The listing builds one solid part. Answer for the finished solid, in the listing's coordinates (mm). Face numbers are marked on the shaded views. A direction names the side the tool comes from. Round coordinates to 2 decimals unless told otherwise and drop trailing zeros. Loops run counter-clockwise (first coordinate to the right, second up) from the corner with the lowest first, then second, coordinate; pieces in that order, holes last. Notation, with made-up numbers: (74, 31.5) -> (93, 31.5) arc R18 ccw to (93, 55.5) -> close; hole circle Ø7 at (-21.5, -1). An arc over 180 degrees is marked (long way). Write each question's results on one line, items separated by ' | '. Start each with the question number.
(1) For the marked faces 1 and 2, determine the directions among +Z, -Z, +X, -X, +Y, -Y from which every point of the face is accessible in a straight line to the end or side of a thin tool.
(2) A straight line is drawn through the part: probe 1 along X at (y, z) = (4.5, 12). Find the intervals that lie inside material, in ascending order.
(3) The part is cut by section A-A (z = 12.5). Determine the outline of the cut face in (x, y), plus the area to 3 significant figures.
(4) The part is cut by section B-B (y = 21.5). Determine the outline of the cut face in (x, z).
```python
from build123d import *

# Parameters (mm, degrees)
SKETCH1_W           = 120
SKETCH1_H           = 34
BOSS_EXTRUDE1_DEPTH = 25
BOSS_EXTRUDE2_DEPTH = 2


with BuildPart() as part:
    # Sketch1 → Boss-Extrude1 (new body)
    with BuildSketch(Plane(origin=(0, 0, 0), x_dir=(1, 0, 0), z_dir=(0, 1, 0))):
        Rectangle(SKETCH1_W, SKETCH1_H)
    extrude(amount=BOSS_EXTRUDE1_DEPTH)

    # Sketch2 → Boss-Extrude2 (add)
    with BuildSketch(Plane.ZY.offset(60)):
        Polygon((8.280528472, 10.841133841), (5.608754496, 18.760489421), (-2.585495606, 20.406343074), (-8.107971731, 14.132841147), (-5.436197754, 6.213485568), (2.758052347, 4.567631915), align=None)
    extrude(amount=BOSS_EXTRUDE2_DEPTH)


solid = part.part
```
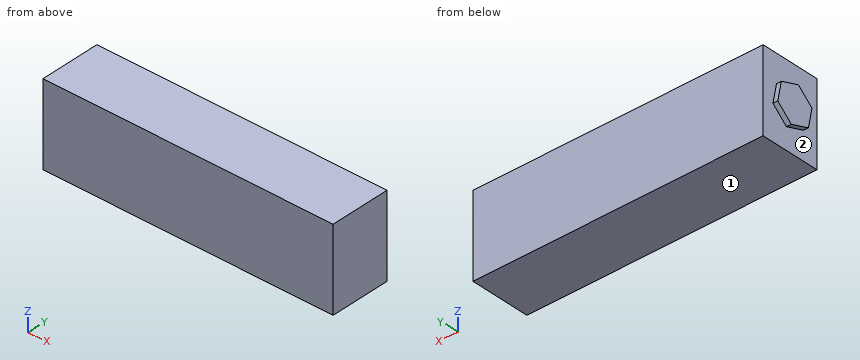
Checked values:
1) face 1: -Z, +X, -X, +Y, -Y | face 2: -X
2) probe 1: x = -60 to 60
3) outline: (-60, 0) -> (60, 0) -> (60, 25) -> (-60, 25) -> close | area: 3,000 mm2
4) outline: (-60, -17) -> (60, -17) -> (60, 17) -> (-60, 17) -> close
